The listing builds one solid part. Answer for the finished solid, in the listing's coordinates (mm). A direction names the side the tool comes from. Give positions to 0.01 mm unless a question says otherwise; leave off trailing zeros. Order: outer loops, then holes, each group sorted by start corner. A loop starts at its lowest first (then second) coordinate and runs counter-clockwise, first axis right, second up.
```python
from build123d import *

# Parameters (mm, degrees)
SKETCH1_R           = 175
BOSS_EXTRUDE1_DEPTH = 30
SKETCH2_R           = 25
SKETCH2_R_2         = 12
BOSS_EXTRUDE2_DEPTH = 50
SKETCH3_R           = 57.5
SKETCH3_R_2         = 54
CUT_EXTRUDE1_DEPTH  = 10


with BuildPart() as part:
    # Sketch1 → Boss-Extrude1 (new body)
    with BuildSketch(Plane(origin=(0, 0, 0), x_dir=(1, 0, 0), z_dir=(0, 1, 0))):
        with Locations(Location((0, 0, 0), (0, 0, 270))):
            Circle(SKETCH1_R)
    extrude(amount=BOSS_EXTRUDE1_DEPTH)

    # Sketch2 → Boss-Extrude2 (add)
    with BuildSketch(Plane(origin=(0, 30, 0), x_dir=(1, 0, 0), z_dir=(0, 1, 0))):
        with Locations(Location((0, 0, 0), (0, 0, 270))):
            Circle(SKETCH2_R)
        with Locations(Location((0, 0, 0), (0, 0, 270))):
            Circle(SKETCH2_R_2, mode=Mode.SUBTRACT)
    extrude(amount=BOSS_EXTRUDE2_DEPTH)

    # Sketch3 → Cut-Extrude1 (cut)
    with BuildSketch(Plane(origin=(0, 30, 0), x_dir=(1, 0, 0), z_dir=(0, 1, 0))):
        with Locations(Location((0, 0, 0), (0, 0, 270))):
            Circle(SKETCH3_R)
        with Locations(Location((0, 0, 0), (0, 0, 270))):
            Circle(SKETCH3_R_2, mode=Mode.SUBTRACT)
    extrude(amount=-CUT_EXTRUDE1_DEPTH, mode=Mode.SUBTRACT)


solid = part.part
```
1) A tool of negligible diameter and unlimited length cuts with its end or side. For faces 4 (the flat face through (6, 80, 11)), 5 (the cylindrical face through (7.509, 54.65, 23.846)), from which of +Z, -Z, +X, -X, +Y, -Y can it reach the whole face along a straight path? Write none if from no direction.
Geometry says:
face 4: +Z, -Z, +X, -X, +Y
face 5: +Y
2) For a pull along X with two mould halves and no side action, classify faces 1 (the flat face through (2, 0, -2)), 2 (the flat face through (0, 30, 0)), 3 (the cylindrical face through (173.51, 14.79, -22.78)) as +X half, -X half, draft (parallel to the pull), parting line (faces both ways), or undercut.
Geometry says:
face 1: draft
face 2: undercut
face 3: parting line
3) Find section D-D (y = 71.5). Write down the section's boundary in (x, z), then the cut area to 3 significant figures.
Geometry says:
outline: circle Ø50 at (0, 0); hole circle Ø24 at (0, 0)
area: 1,510 mm2
4) Find section C-C (y = 7). Write down the section's boundary in (x, z), then the cut area to 3 significant figures.
Geometry says:
outline: circle Ø350 at (0, 0)
area: 96,200 mm2
5) Find section B-B (z = 0). Write down the section's boundary in (x, y), then the cut area to 3 significant figures.
Geometry says:
outline: (-175, 0) - (175, 0) - (175, 30) - (57.5, 30) - (57.5, 20) - (54, 20) - (54, 30) - (25, 30) - (25, 80) - (12, 80) - (12, 30) - (-12, 30) - (-12, 80) - (-25, 80) - (-25, 30) - (-54, 30) - (-54, 20) - (-57.5, 20) - (-57.5, 30) - (-175, 30) - close
area: 11,700 mm2
6) Find section A-A (x = -44). Write down the section's boundary in (y, z).
Geometry says:
outline: (0, -169.38) - (30, -169.38) - (30, -37.02) - (20, -37.02) - (20, -31.3) - (30, -31.3) - (30, 31.3) - (20, 31.3) - (20, 37.02) - (30, 37.02) - (30, 169.38) - (0, 169.38) - close
7) Given P1, Ø2, axis at y = 20.5, z = -49, coming from the -X side; P2, Ø5, axis at x = 109.5, y = 23.5, coming from the +Z side; P3, Ø1.5, axis at x = -71, y = 8.5, coming from the +Z side, each flat-ended and moving along its own axis, determine where each tip first touches the part or whether it passes through.
Geometry says:
P1: stops at x = -168.29
P2: stops at z = 138.48
P3: stops at z = 160.28
8) Straight lines are drawn through the part: probe 1 along X at (y, z) = (23, 0); probe 2 along X at (y, z) = (65.5, 0); probe 3 along Y at (x, z) = (31, -44.5). For each, find the intervals that lie inside material, in ascending order.
Geometry says:
probe 1: x = -175 to -57.5, -54 to 54, 57.5 to 175
probe 2: x = -25 to -12, 12 to 25
probe 3: y = 0 to 20
